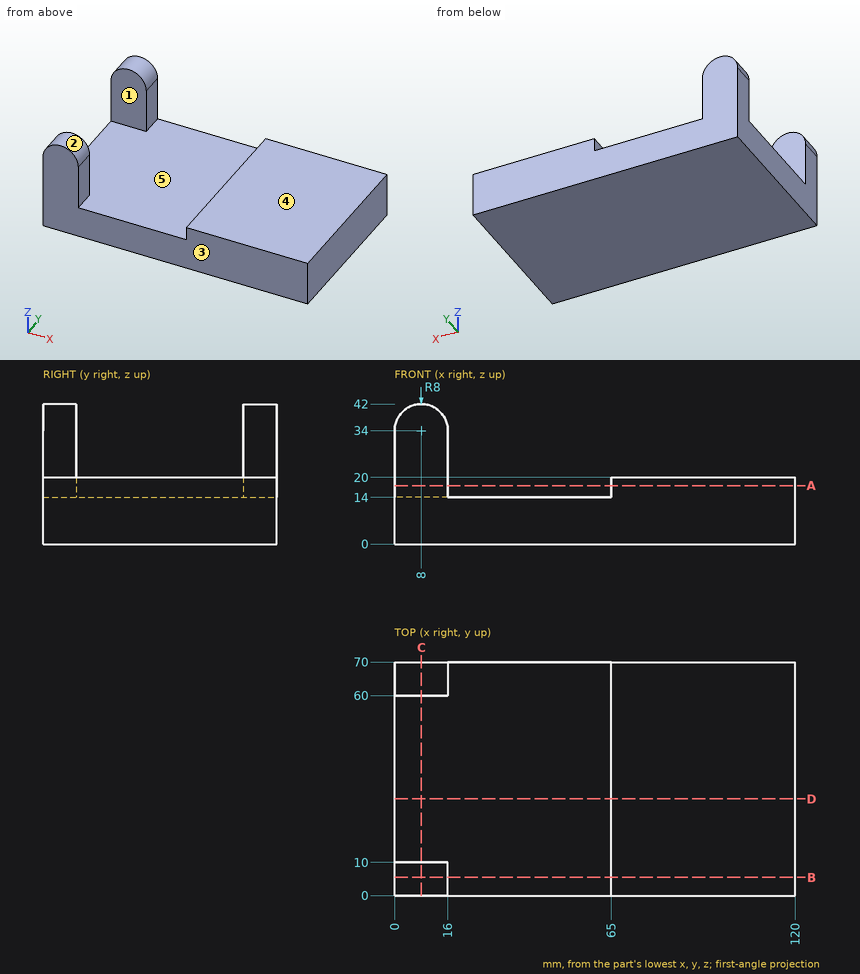
Here's the drawing with two shaded views (mm, measured from the low corner). I have some questions. A direction names the side the tool comes from. Give positions to 0.01 mm unless a question says otherwise; leave off trailing zeros. Order: outer loops, then holes, each group sorted by start corner. A loop starts at its lowest first (then second) coordinate and runs counter-clockwise, first axis right, second up. Notation, with made-up numbers: M 88.5,-15.5 L 132.5,-15.5 A19 cw 132.5,15.5 Z; hole C 40,23.25 d5. An arc over 180 degrees is marked long. Answer as a JSON object with one key per item and string values. Group by question number.
1) Suppose I cut it at B-B, the plane y = 5.5. Write out the boundary of the cut face in (x, z), plus the area to 3 significant figures.
2) I'm going to push flat-ended pins straight in: pin 1 Ø16.5 at (x, y) = (85, 52.5) entering from +Z; pin 2 Ø6.5 at (y, z) = (50.5, 16) entering from -X; pin 3 Ø6 at (y, z) = (9.5, 28.5) entering from +X. Where does each tip first touch, or does it pass through?
3) On a 3-axis mill with a long thin cutter (end or side, diameter ignored), from which of +Z, -Z, +X, -X, +Y, -Y can I reach the whole of each face in a straight line? I mean the marked faces 1 and 2. Say none if no direction works.
4) Please list where these lines run through material, in increasing order: L1, parallel to Y at x = 11.5, z = 27.5; L2, parallel to X at y = 9, z = 18.5; L3, parallel to Z at x = 37, y = 7.5. Write a range as [from, to].
5) Suppose I cut it at C-C, the plane x = 8. Write out the boundary of the cut face in (y, z).
6) Suppose I cut it at A-A, the plane z = 17.5. Write out the boundary of the cut face in (x, y), plus the area to 3 significant figures.
7) Suppose I cut it at D-D, the plane y = 29. Write out the boundary of the cut face in (x, z).
8) We'd pull the mould along Y, two halves only. Please class the marked faces 3, 4 and 5: pulls with the +Y half, pulls with the -Y half, needs draft (parallel to the pull), parting line crosses it, or undercut.
Results found:
{
 "1": {"outline": "M 0,0 L 120,0 L 120,20 L 65,20 L 65,14 L 16,14 L 16,34 A8 ccw 0,34 Z", "area": "2,430 mm²"},
 "2": {"pin 1": "z = 20", "pin 2": "x = 0", "pin 3": "x = 16"},
 "3": {"face 1": "+Z, -X", "face 2": "+Z, +Y, -Y"},
 "4": {"L1": "[0, 10], [60, 70]", "L2": "[0, 16], [65, 120]", "L3": "[0, 14]"},
 "5": {"outline": "M 0,0 L 70,0 L 70,42 L 60,42 L 60,14 L 10,14 L 10,42 L 0,42 Z"},
 "6": {"outline": "M 0,0 L 16,0 L 16,10 L 0,10 Z; M 0,60 L 16,60 L 16,70 L 0,70 Z; M 65,0 L 120,0 L 120,70 L 65,70 Z", "area": "4,170 mm²"},
 "7": {"outline": "M 0,0 L 120,0 L 120,20 L 65,20 L 65,14 L 0,14 Z"},
 "8": {"face 3": "pulls with the -Y half", "face 4": "needs draft", "face 5": "undercut"}
}
